Build history of the part. All positions in model axes, mm. A direction names the side the tool comes from. Give positions to 0.01 mm unless a question says otherwise; leave off trailing zeros. Write each loop counter-clockwise with the first axis right and the second up, starting at its lowest first coordinate (ties: lowest second). Pieces come first, ordered by that corner, then holes.
from build123d import *

# Parameters (mm, degrees)
SKETCH1_R               = 5.5626
BOSS_EXTRUDE1_DEPTH     = 55.5244
CUT_EXTRUDE1_DEPTH      = 57.078908984
CUT_EXTRUDE1_DEPTH_BACK = 57.078908984
SKETCH2_R               = 1.6256
CUT_EXTRUDE2_DEPTH      = 57.078909103
CUT_EXTRUDE2_DEPTH_BACK = 57.078909103
SKETCH3_W               = 4.7498
SKETCH3_H               = 17.4244


with BuildPart() as part:
    # Sketch1 → Boss-Extrude1 (new body)
    with BuildSketch(Plane(origin=(0, 0, 0), x_dir=(1, 0, 0), z_dir=(0, 1, 0))):
        with Locations(Location((0, 0, 0), (0, 0, 90))):
            Circle(SKETCH1_R)
    extrude(amount=BOSS_EXTRUDE1_DEPTH)

    # Sketch2 → Cut-Extrude1 (cut, two sides: drawn at the far end of the back side and taken through both)
    with BuildSketch(Plane.XY.offset(-CUT_EXTRUDE1_DEPTH_BACK)):
        with Locations(Location((0, 50.7619, 0), (0, 0, 89.999999974))):
            Circle(SKETCH2_R)
    extrude(amount=CUT_EXTRUDE1_DEPTH + CUT_EXTRUDE1_DEPTH_BACK, mode=Mode.SUBTRACT)

    # Sketch3 → Cut-Extrude2 (cut, two sides: drawn at the far end of the back side and taken through both)
    with BuildSketch(Plane(origin=(0, 0, 0), x_dir=(0, 0, -1), z_dir=(1, 0, 0)).offset(-CUT_EXTRUDE2_DEPTH_BACK)):
        with Locations((0, 46.8122)):
            Rectangle(SKETCH3_W, SKETCH3_H)
    extrude(amount=CUT_EXTRUDE2_DEPTH + CUT_EXTRUDE2_DEPTH_BACK, mode=Mode.SUBTRACT)


solid = part.part
1. Drop flat-ended pins along their axis: pin 1 (4 mm diameter, centred on y = 45, z = 4, fed in from -X); pin 2 (1.4 mm diameter, centred on x = -1.5, z = 0, fed in from +Y); pin 3 (2 mm diameter, centred on y = 11.5, z = 1.5, fed in from +X). Give the stop position or say it passes through.
2. 3-axis set-ups, long thin cutter, end or side, ignore diameter. For faces 4 (the face through (0, 38.1, 0)), 5 (the face through (-0.49, 52.31, 3.95)): which of +Z, -Z, +X, -X, +Y, -Y reach the whole face in a straight line?
3. Mould opens along Z. For faces 1 (the face through (0, 47, 2.375)), 2 (the face through (0, 0, 0)), 3 (the face through (-1.671, 27.374, -5.306)) say: pulls with the +Z half, pulls with the -Z half, needs draft (parallel to the pull), parting line crosses it, or undercut.
4. Saw through at A-A on x = 0. Give the cut face in (y, z).
5. Saw through at D-D on x = 3.25. Give the cut face in (y, z).
6. Drill centre lines: line 1 along Y through (x, z) = (-3.75, -0.75); line 2 along Z through (x, y) = (1.5, 45.5); line 3 along Z through (x, y) = (0.75, 46). Where is each one in solid material? Low to high.
7. Saw through at C-C on z = -4.5. Give the cut face in (x, y), plus the area to 3 significant figures.
8. Saw through at B-B on y = 43. Give the cut face in (x, z).
Outcome:
1. pin 1: stops at x = -5.03
1. pin 2: stops at y = 38.1
1. pin 3: stops at x = 5.54
2. face 4: +X, -X, +Y
2. face 5: +Z, -Z
3. face 1: undercut
3. face 2: needs draft
3. face 3: parting line crosses it
4. outline: (0, -5.56) - (49.14, -5.56) - (49.14, -2.37) - (38.1, -2.37) - (38.1, 2.37) - (49.14, 2.37) - (49.14, 5.56) - (0, 5.56) - close; (52.39, -5.56) - (55.52, -5.56) - (55.52, -2.37) - (52.39, -2.37) - close; (52.39, 2.37) - (55.52, 2.37) - (55.52, 5.56) - (52.39, 5.56) - close
5. outline: (0, -4.51) - (55.52, -4.51) - (55.52, -2.37) - (38.1, -2.37) - (38.1, 2.37) - (55.52, 2.37) - (55.52, 4.51) - (0, 4.51) - close
6. line 1: y = 0 to 38.1
6. line 2: z = -5.36 to -2.37, 2.37 to 5.36
6. line 3: z = -5.51 to -2.37, 2.37 to 5.51
7. outline: (-3.27, 0) - (3.27, 0) - (3.27, 55.52) - (-3.27, 55.52) - close; hole circle Ø3.25 at (0, 50.76)
7. area: 355 mm2
8. outline: (-5.03, -2.37) arc R5.56 ccw to (5.03, -2.37) - close; (-5.03, 2.37) - (5.03, 2.37) arc R5.56 ccw to start
